from build123d import *

# Parameters (mm, degrees)
SKETCH1_W               = 30.562599784
SKETCH1_H               = 30.562599784
BOSS_EXTRUDE1_DEPTH     = 139.7
CUT_EXTRUDE1_DEPTH      = 142.361685943
CUT_EXTRUDE1_DEPTH_BACK = 142.361685943
BOSS_EXTRUDE2_DEPTH     = 5.09983
SKETCH5_R               = 1.8
CUT_EXTRUDE2_DEPTH      = 146.354775845
SKETCH6_R               = 1.662500104
CUT_EXTRUDE3_DEPTH      = 145.138064655


with BuildPart() as part:
    # Sketch1 → Boss-Extrude1 (new body)
    with BuildSketch(Plane(origin=(0, 0, 0), x_dir=(1, 0, 0), z_dir=(0, 1, 0))):
        Rectangle(SKETCH1_W, SKETCH1_H)
    extrude(amount=BOSS_EXTRUDE1_DEPTH)

    # Sketch2 → Cut-Extrude1 (cut, two sides: drawn at the far end of the back side and taken through both)
    with BuildSketch(Plane(origin=(0, 0, 0), x_dir=(0.7071067811865477, 0, -0.7071067811865475), z_dir=(0.7071067811865475, 0, 0.7071067811865477)).offset(-CUT_EXTRUDE1_DEPTH_BACK)):
        Polygon((5.11931044, 139.7), (0, 81.186013921), (21.611021558, 79.295294527), (21.611021558, 139.7), align=None)
    extrude(amount=CUT_EXTRUDE1_DEPTH + CUT_EXTRUDE1_DEPTH_BACK, mode=Mode.SUBTRACT)

    # Sketch4 → Boss-Extrude2 (add)
    with BuildSketch(Plane(origin=(-4.984326181, 0.616698988, 4.984326181), x_dir=(-0.6990853645605906, 0.08649619246092877, -0.7097873355780225), z_dir=(0.704416026402759, -0.08715574274765817, -0.7044160264027586))):
        Polygon((-16.344826658, 141.568383735), (40.589342943, 136.606243895), (35.627203104, 79.672074294), (-21.306966498, 84.634214133), align=None)
    extrude(amount=-BOSS_EXTRUDE2_DEPTH)

    # Sketch5 → Cut-Extrude2 (cut, through all)
    with BuildSketch(Plane(origin=(-4.984326181, 0.616698988, 4.984326181), x_dir=(-0.6990853645605907, 0.08649619246092867, -0.7097873355780224), z_dir=(0.7044160264027588, -0.08715574274765812, -0.7044160264027586))):
        with Locations(Location((33.963841811, 130.554186497, 0), (0, 0, 355.018930606))):
            Circle(SKETCH5_R)
        with Locations(Location((-10.866212993, 134.461383221, 0), (0, 0, 355.018930606))):
            Circle(SKETCH5_R)
        with Locations(Location((-14.773409717, 89.631328416, 0), (0, 0, 355.018930606))):
            Circle(SKETCH5_R)
        with Locations(Location((30.056645087, 85.724131693, 0), (0, 0, 355.018930606))):
            Circle(SKETCH5_R)
        Polygon((19.712476114, 122.520420225), (9.750241713, 123.388686164), (9.22928215, 117.411345523), (19.191516551, 116.543079585), align=None)
    extrude(amount=-CUT_EXTRUDE2_DEPTH, mode=Mode.SUBTRACT)

    # Sketch6 → Cut-Extrude3 (cut, symmetric)
    with BuildSketch(Plane(origin=(0, 0, 0), x_dir=(0, 0, -1), z_dir=(1, 0, 0))):
        with Locations(Location((0, 25.4, 0), (0, 0, 180))):
            Circle(SKETCH6_R)
        with Locations(Location((-9.5, 15.9, 0), (0, 0, 180))):
            Circle(SKETCH6_R)
        with Locations(Location((9.5, 15.9, 0), (0, 0, 180))):
            Circle(SKETCH6_R)
        with Locations(Location((0, 6.4, 0), (0, 0, 180))):
            Circle(SKETCH6_R)
    cut_extrude3 = extrude(amount=CUT_EXTRUDE3_DEPTH, both=True, mode=Mode.SUBTRACT)

    # Mirror1: Cut-Extrude3 across plane
    add(cut_extrude3.mirror(Plane(origin=(0, 0, 0), x_dir=(-0.7071067811865478, 0, 0.7071067811865472), z_dir=(0.7071067811865475, 0, 0.7071067811865477))), mode=Mode.SUBTRACT)


solid = part.part
Can you work these out from the model? Positions are in its coordinate system, mm. A direction names the side the tool comes from. Coordinates: 2 decimals unless noted, no trailing zeros. Order: outer loops, then holes, each group sorted by start corner. A loop starts at its lowest first (then second) coordinate and runs counter-clockwise, first axis right, second up. Notation, with made-up numbers: (-33.5, 39) - (13.5, 39) arc R17 cw to (13.5, 57) - close; hole circle Ø5 at (67, 74). An arc over 180 degrees is marked (long way). Answer as a JSON object with one key per item and string values. Group by question number.
Q1. Will these pins go through, and if not, where does the flat tip stop? P1, Ø8, axis at x = -11, y = 56, coming from the +Z side; P2, Ø9, axis at y = 84, z = 1, coming from the -X side; P3, Ø1.5, axis at x = -2, z = -3.5, coming from the +Y side.
Q2. On a 3-axis mill with a long thin cutter (end or side, diameter ignored), from which of +Z, -Z, +X, -X, +Y, -Y can I reach the whole of each face in a straight line? I mean faces 5 (the face through (5.622, 80.464, -6.05)), 6 (the face through (0, 40, -15.281)), 7 (the face through (-7.08, 124.76, 1.32)), 8 (the face through (-10.4, 14.5, -13)), 9 (the face through (-13, 14.5, -8.6)). Say none if no direction works.
Q3. Imagine slicing it at B-B (x = 5.5). Please give me the cut outline in (y, z) (1 decimal), and give its area (3 significant figures).
Q4. We'd pull the mould along X, two halves only. Please class faces 1 (the face through (-5.32, 122.018, 6.734)), 2 (the face through (20.27, 111.05, 20.14)), 3 (the face through (7.748, 26.037, 1.536)), 4 (the face through (-15.764, 104.32, -11.386)): +X half, -X half, draft (parallel to the pull), parting line (faces both ways), or undercut.
Q5. Imagine slicing it at C-C (y = 55.5). Please give me the cut outline in (x, z).
Q6. I need wall thicknesses on line 1 (X direction, y = 15.9, z = -13.7); line 2 (Y direction, x = -12, z = 9). Which ranges of each line are inside material? Lowest first, please. Write a range as from..to.
Q7. Imagine slicing it at A-A (y = 6.4). Please give me the cut outline in (x, z).
Determined:
{
 "1": {"P1": "stops at z = 15.28", "P2": "stops at x = -15.28", "P3": "stops at y = 140.12"},
 "2": {"face 5": "-Z, +X", "face 6": "-Z, +X, -X, -Y", "face 7": "none", "face 8": "+Z, -Z", "face 9": "+X, -X"},
 "3": {"outline": "(0, -15.3) - (79.9, -15.3) - (81.2, 5.5) - (139.7, -1.7) - (140.1, 5.4) - (139.7, 5.5) - (139.7, 15.3) - (0, 15.3) - close; hole circle Ø3.3 at (6.4, 0); hole circle Ø3.3 at (15.9, -9.5); hole circle Ø3.3 at (15.9, 9.5); hole circle Ø3.3 at (25.4, 0)", "area": "3,220 mm2"},
 "4": {"face 1": "undercut", "face 2": "+X half", "face 3": "draft", "face 4": "-X half"},
 "5": {"outline": "(-15.28, -15.28) - (15.28, -15.28) - (15.28, 15.28) - (-15.28, 15.28) - close"},
 "6": {"line 1": "x = -15.28..-11.16, -7.84..7.84, 11.16..15.28", "line 2": "y = 0..14.31, 17.49..119.52, 125.54..139.7"},
 "7": {"outline": "(-15.28, -15.28) - (-1.66, -15.28) - (-1.66, -1.66) - (-15.28, -1.66) - close; (-15.28, 1.66) - (-1.66, 1.66) - (-1.66, 15.28) - (-15.28, 15.28) - close; (1.66, -15.28) - (15.28, -15.28) - (15.28, -1.66) - (1.66, -1.66) - close; (1.66, 1.66) - (15.28, 1.66) - (15.28, 15.28) - (1.66, 15.28) - close"}
}
